For this review, take the finished solid that the model builds, in its own axes (mm). A direction names the side the tool comes from. Round coordinates to 2 decimals unless told otherwise and drop trailing zeros. Loops run counter-clockwise (first coordinate to the right, second up) from the corner with the lowest first, then second, coordinate; pieces in that order, holes last. Notation, with made-up numbers: (-25, -38) -> (-9, -38) arc R18 ccw to (-9, -34) -> close; hole circle Ø10 at (33, 30). An arc over 180 degrees is marked (long way). Write each question's results on one line, items separated by ' | '.
```python
from build123d import *

# Parameters (mm, degrees)
BOSS_EXTRUDE1_OUTLINE_R = 1.75
BOSS_EXTRUDE1_DEPTH     = 4
SKETCH2_W               = 0.569871795
SKETCH2_H               = 3.175
CUT_EXTRUDE1_DEPTH      = 1


# Read off the part's stored shape, not the designer's step: Boss-Extrude1
with BuildPart() as part:
    # Boss-Extrude1 outline → Boss-Extrude1 (new body)
    with BuildSketch(Plane(origin=(0, 0, 0), x_dir=(1, 0, 0), z_dir=(0, 1, 0))):
        with BuildLine():
            Line((25.296474615, -10.33744254), (37.54307775, -10.33744254))
            ThreePointArc((37.54307775, -10.33744254), (39.979776182, -5.587442326), (42.416474615, -10.33744254))
            Line((42.416474615, -10.33744254), (49.479776182, -10.33744254))
            Line((49.479776182, -10.33744254), (49.479776182, -18.81631662))
            Line((49.479776182, -18.81631662), (58.579776182, -18.81631662))
            Line((58.579776182, -18.81631662), (58.579776182, -4.977921711))
            Line((58.579776182, -4.977921711), (-21.420223818, -4.977921711))
            Line((-21.420223818, -4.977921711), (-21.420223818, -18.81631662))
            Line((-21.420223818, -18.81631662), (-12.320223818, -18.81631662))
            Line((-12.320223818, -18.81631662), (-12.320223818, -10.33744254))
            Line((-12.320223818, -10.33744254), (3.30307775, -10.33744254))
            ThreePointArc((3.30307775, -10.33744254), (5.739776182, -5.587442326), (8.176474615, -10.33744254))
            Line((8.176474615, -10.33744254), (20.42307775, -10.33744254))
            ThreePointArc((20.42307775, -10.33744254), (22.859776182, -5.587442326), (25.296474615, -10.33744254))
        make_face()
        with Locations((-16.420223818, -13.587442433)):
            Circle(BOSS_EXTRUDE1_OUTLINE_R, mode=Mode.SUBTRACT)
        with Locations((53.579776182, -13.587442433)):
            Circle(BOSS_EXTRUDE1_OUTLINE_R, mode=Mode.SUBTRACT)
    extrude(amount=BOSS_EXTRUDE1_DEPTH)

    # Sketch2 → Cut-Extrude1 (cut)
    with BuildSketch(Plane(origin=(0, 4, 0), x_dir=(1, 0, 0), z_dir=(0, 1, 0))):
        Polygon((-18.749121586, -7.085274104), (-17.202326714, -7.085274104), (-17.202326714, -7.655145899), (-18.179249791, -7.655145899), (-18.179249791, -8.265722822), (-17.202326714, -8.265722822), (-17.202326714, -8.835594617), (-18.179249791, -8.835594617), (-18.179249791, -10.260274104), (-18.749121586, -10.260274104), align=None)
        Polygon((-16.826440296, -7.085274104), (-16.15480568, -7.085274104), (-15.491439294, -8.104810362), (-14.826800873, -7.085274104), (-14.153258204, -7.085274104), (-15.154985969, -8.621256676), (-14.088384406, -10.260274104), (-14.760019022, -10.260274104), (-15.491439294, -9.136430955), (-16.224131602, -10.260274104), (-16.897038253, -10.260274104), (-15.827256602, -8.619984641), align=None)
        with Locations((-13.45745492, -8.672774104)):
            Rectangle(SKETCH2_W, SKETCH2_H)
    extrude(amount=-CUT_EXTRUDE1_DEPTH, mode=Mode.SUBTRACT)


solid = part.part
```
1. Draft analysis for pull direction X (two halves, no side actions). For faces 4 (the face through (19, 2, 4.978)), 5 (the face through (22.77, 1.97, 5.59)), 6 (the face through (-21.42, 2, 12)), state which applies: released by +X, released by -X, zero draft, split by the parting line, or undercut.
Values found:
face 4: zero draft | face 5: undercut | face 6: released by -X
2. Tool access review of faces 1 (the face through (31, 2, 10.337)), 2 (the face through (-15.5, 3, 8.7)), 3 (the face through (39.89, 1.97, 5.59)): name each direction out of +Z, -Z, +X, -X, +Y, -Y from which nothing blocks a thin tool from reaching the whole face with its end or side.
Values found:
face 1: +Z, +Y, -Y | face 2: +Y | face 3: +Y, -Y
3. Consider section C-C (x = 7.5). State the section outline as (y, z) points, plus the area to 3 significant figures.
Values found:
outline: (0, 4.98) -> (4, 4.98) -> (4, 6.16) -> (0, 6.16) -> close | area: 4.72 mm2
4. Consider section D-D (x = -9). State the section outline as (y, z) points, plus the area to 3 significant figures.
Values found:
outline: (0, 4.98) -> (4, 4.98) -> (4, 10.34) -> (0, 10.34) -> close | area: 21.4 mm2
5. Consider section B-B (y = 0.6). State the section outline as (x, z) points, plus the area to 3 significant figures.
Values found:
outline: (-21.42, 4.98) -> (58.58, 4.98) -> (58.58, 18.82) -> (49.48, 18.82) -> (49.48, 10.34) -> (42.42, 10.34) arc R3 cw (long way) to (37.54, 10.34) -> (25.3, 10.34) arc R3 cw (long way) to (20.42, 10.34) -> (8.18, 10.34) arc R3 cw (long way) to (3.3, 10.34) -> (-12.32, 10.34) -> (-12.32, 18.82) -> (-21.42, 18.82) -> close; hole circle Ø3.5 at (-16.42, 13.59); hole circle Ø3.5 at (53.58, 13.59) | area: 492 mm2
6. For pin 1 (1.5 mm diameter, centred on x = 14.5, y = 0.5, fed in from +Z), flat-tipped, find the tip position at first contact; note if it passes through.
Values found:
pin 1: stops at z = 10.34
7. To check wall thickness, follow probe 1 along X at (y, z) = (3.2, 16); probe 2 along X at (y, z) = (1.9, 14.5); probe 3 along X at (y, z) = (0.55, 13). State the ranges of each line that lie inside material, in increasing order.
Values found:
probe 1: x = -21.42 to -12.32, 49.48 to 58.58 | probe 2: x = -21.42 to -17.91, -14.93 to -12.32, 49.48 to 52.09, 55.07 to 58.58 | probe 3: x = -21.42 to -18.07, -14.77 to -12.32, 49.48 to 51.93, 55.23 to 58.58
8. Consider section A-A (z = 16.5). State the section outline as (x, y) points.
Values found:
outline: (-21.42, 0) -> (-12.32, 0) -> (-12.32, 4) -> (-21.42, 4) -> close; (49.48, 0) -> (58.58, 0) -> (58.58, 4) -> (49.48, 4) -> close
